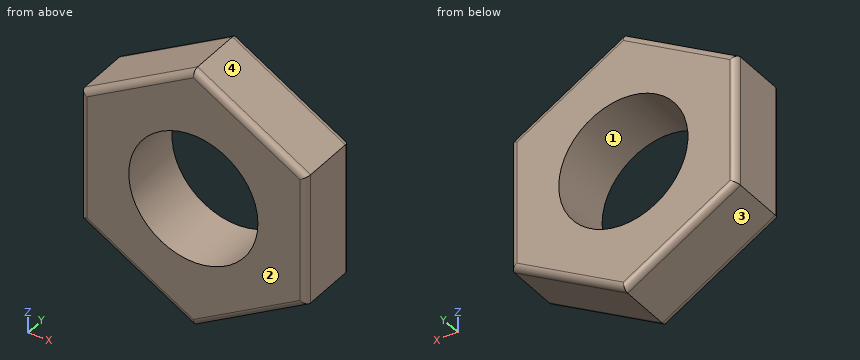
```python
from build123d import *

# Parameters (mm, degrees)
BOSS_EXTRUDE1_DEPTH      = 2
F_4_0_4_DIAMETER_HOLE1_D = 4
FILLET1_R                = 0.2


with BuildPart() as part:
    # Sketch1 → Boss-Extrude1 (new body)
    with BuildSketch(Plane(origin=(0, 2, 0), x_dir=(1, 0, 0), z_dir=(0, 1, 0))):
        Polygon((0, 4.041451884), (-3.5, 2.020725942), (-3.5, -2.020725942), (0, -4.041451884), (3.5, -2.020725942), (3.5, 2.020725942), align=None)
    extrude(amount=-BOSS_EXTRUDE1_DEPTH)

    # Ø4.0 (4) Diameter Hole1 (through all)
    with Locations(Plane(origin=(0, 0, 0), x_dir=(-1, 0, 0), z_dir=(0, -1, 0))):
        with Locations((0, 0)):
            Hole(F_4_0_4_DIAMETER_HOLE1_D / 2)

    # Fillet1
    fillet1_edges = [part.edges().sort_by_distance(p)[0] for p in [
        (-3.5, 0, 0),
        (-1.75, 0, 3.031088913),
        (1.75, 0, 3.031088913),
        (3.5, 0, 0),
        (1.75, 0, -3.031088913),
        (3.5, 2, 0),
        (1.75, 2, 3.031088913),
        (-1.75, 2, 3.031088913),
        (-3.5, 2, 0),
        (-1.75, 2, -3.031088913),
        (1.75, 2, -3.031088913),
        (-1.75, 0, -3.031088913),
    ]]
    fillet(fillet1_edges, radius=FILLET1_R)


solid = part.part
```
Here's how the part is built. I have some questions about the finished solid (model axes, mm). Face numbers are marked on the shaded views. Round coordinates to 2 decimals unless told otherwise and drop trailing zeros. Write each loop counter-clockwise with the first axis right and the second up, starting at its lowest first coordinate (ties: lowest second). Pieces come first, ordered by that corner, then holes.
Q1. If we section it at B-B on y = 1.35: Write out the boundary of the cut face in (x, z).
Q2. If we section it at C-C on z = 1.5: Write out the boundary of the cut face in (x, y).
Q3. If we mould it in two halves opening along Z, with no side actions, what happens to the marked faces 1, 2, 3 and 4? For each: +Z half, -Z half, draft (parallel to the pull), parting line (faces both ways), or undercut.
Q4. If we section it at A-A on z = 0: Write out the boundary of the cut face in (x, y).
Q5. Please list where these lines run through material, in increasing order: probe 1 along X at (y, z) = (1.9, -1.5); probe 2 along Z at (x, y) = (-1.5, 0.4); probe 3 along Z at (x, y) = (0.5, 1.4).
Answer below:
1. outline: (-3.5, -2.02) - (0, -4.04) - (3.5, -2.02) - (3.5, 2.02) - (0, 4.04) - (-3.5, 2.02) - close; hole circle Ø4 at (0, 0)
2. outline: (-3.5, 0.2) arc R0.2 ccw to (-3.3, 0) - (-1.32, 0) - (-1.32, 2) - (-3.3, 2) arc R0.2 ccw to (-3.5, 1.8) - close; (1.32, 0) - (3.3, 0) arc R0.2 ccw to (3.5, 0.2) - (3.5, 1.8) arc R0.2 ccw to (3.3, 2) - (1.32, 2) - close
3. face 1: undercut
3. face 2: draft
3. face 3: -Z half
3. face 4: +Z half
4. outline: (-3.5, 0.2) arc R0.2 ccw to (-3.3, 0) - (-2, 0) - (-2, 2) - (-3.3, 2) arc R0.2 ccw to (-3.5, 1.8) - close; (2, 0) - (3.3, 0) arc R0.2 ccw to (3.5, 0.2) - (3.5, 1.8) arc R0.2 ccw to (3.3, 2) - (2, 2) - close
5. probe 1: x = -3.47 to -1.32, 1.32 to 3.47
5. probe 2: z = -3.18 to -1.32, 1.32 to 3.18
5. probe 3: z = -3.75 to -1.94, 1.94 to 3.75
